Input: part model. Units: mm. Frame: model coordinates. A direction names the side the tool comes from. Give positions to 0.01 mm unless a question says otherwise; leave off trailing zeros. Loops run counter-clockwise (first coordinate to the right, second up) from the corner with the lowest first, then second, coordinate; pieces in that order, holes last. Notation, with made-up numbers: M 0,7.25 L 33,7.25 A14 ccw 33,32.25 Z; hole C 22.25,-8.5 d5. An arc over 180 degrees is marked long. Use CSV: the item, a comma, the result in double quotes. Start each with the question number.
Q1. Reachability of faces 4 (the flat face through (1, 12.573, 6)), 5 (the flat face through (1, 2.286, -1)), 6 (the cylindrical face through (4.34, 46.73, 6.39)) from +Z, -Z, +X, -X, +Y, -Y: full face, straight path, thin tool, end or side. Return the list, or none.
Q2. Section C-C, the plane x = 2. Output: boundary loops of the cut face in (y, z) (3 decimals).
Q3. Pull-direction query (Y, two-part tool) for faces 1 (the cylindrical face through (1.428, 11.809, 9.385)), 2 (the flat face through (18.128, 46, 6)), 3 (the cylindrical face through (1.528, 51.891, 6.386)); classes: released by +Y, released by -Y, zero draft, split by the parting line, or undercut.
Q4. Pin query (flat end, axial travel): pin 1 (0.9 mm diameter, centred on x = 2, z = 7.5, fed in from +Y); pin 2 (8 mm diameter, centred on x = 8.5, y = 11, fed in from -Z); pin 3 (1 mm diameter, centred on x = 1.5, y = 9.5, fed in from -Z); pin 4 (2 mm diameter, centred on x = 9, z = 4, fed in from -Y). Return the tip coordinate at first contact, or that it passes through.
Q5. Section D-D, the plane y = 28. Output: boundary loops of the cut face in (x, z), plus the area to 3 significant figures.
Q6. Section A-A, the plane y = 45.5. Output: boundary loops of the cut face in (x, z), plus the area to 3 significant figures.
Q7. Material intervals for line 1 along Y through (x, z) = (1.5, 5.5) (3 decimals); line 2 along X through (y, z) = (38, 2.5); line 3 along Y through (x, z) = (1, 5.25) (3 decimals), sorted ascending.
Q8. Section B-B, the plane z = 9.25. Output: boundary loops of the cut face in (x, y), plus the area to 3 significant figures.
from build123d import *

# Parameters (mm, degrees)
F1_DEPTH = 12.954
F2_W     = 5.715
F2_H     = 7.2644
F3_DEPTH = 18.129257
F5_DEPTH = 2.8956


with BuildPart() as f1:
    # F0 (on Top) → F1 (new body)
    with BuildSketch(Plane.XY):
        with BuildLine():
            Line((0, 48.26), (0, 0))
            Line((0, 0), (2.8956, 0))
            Line((2.8956, 0), (2.8956, 43.18))
            ThreePointArc((2.8956, 43.18), (4.383498, 46.772102), (7.9756, 48.26))
            Line((7.9756, 48.26), (10.538739, 48.26))
            ThreePointArc((10.538739, 48.26), (13.963674, 46.931829), (15.597704, 43.641818))
            ThreePointArc((15.597704, 43.641818), (15.761106, 43.312817), (16.1036, 43.18))
            Line((16.1036, 43.18), (17.620257, 43.18))
            ThreePointArc((17.620257, 43.18), (17.979467, 43.32879), (18.128257, 43.688))
            Line((18.128257, 43.688), (18.128257, 48.26))
            ThreePointArc((18.128257, 48.26), (16.64036, 51.852102), (13.048257, 53.34))
            Line((13.048257, 53.34), (5.08, 53.34))
            ThreePointArc((5.08, 53.34), (1.487898, 51.852102), (0, 48.26))
        make_face()
    extrude(amount=F1_DEPTH)

    # F2 (on face) → F3 (cut, through all)
    with BuildSketch(Plane(origin=(0, 0, 0), x_dir=(0, -1, 0), z_dir=(-1, 0, 0))):
        with BuildLine():
            ThreePointArc((-15.875, 3.3528), (-15.72621, 2.99359), (-15.367, 2.8448))
            Line((-15.367, 2.8448), (-8.001, 2.8448))
            Line((-8.001, 2.8448), (-8.001, 10.1092))
            Line((-8.001, 10.1092), (-10.033, 10.1092))
            ThreePointArc((-10.033, 10.1092), (-11.829051, 9.365251), (-12.573, 7.5692))
            Line((-12.573, 7.5692), (-12.573, 4.445))
            ThreePointArc((-12.573, 4.445), (-12.72179, 4.08579), (-13.081, 3.937))
            Line((-13.081, 3.937), (-14.351, 3.937))
            ThreePointArc((-14.351, 3.937), (-14.71021, 4.08579), (-14.859, 4.445))
            Line((-14.859, 4.445), (-14.859, 5.842))
            Line((-14.859, 5.842), (-13.97, 5.842))
            Line((-13.97, 5.842), (-13.97, 6.604))
            ThreePointArc((-13.97, 6.604), (-14.11879, 6.96321), (-14.478, 7.112))
            Line((-14.478, 7.112), (-15.367, 7.112))
            ThreePointArc((-15.367, 7.112), (-15.72621, 6.96321), (-15.875, 6.604))
            Line((-15.875, 6.604), (-15.875, 3.3528))
        make_face()
        with Locations((-3.8735, 6.477)):
            Rectangle(F2_W, F2_H)
    extrude(amount=-F3_DEPTH, mode=Mode.SUBTRACT)

    # F4 (on Right) → F5 (join, through all)
    with BuildSketch(Plane.YZ):
        with BuildLine():
            Line((2.286, 0), (0, 0))
            Line((0, 0), (0, -1.524))
            ThreePointArc((0, -1.524), (0.371974, -2.422026), (1.27, -2.794))
            Line((1.27, -2.794), (2.286, -2.794))
            Line((2.286, -2.794), (2.286, 0))
        make_face()
    extrude(amount=F5_DEPTH)


solid = f1.part
A:
1,face 4,"+X, -X"
1,face 5,"-Z, +X, -X, +Y"
1,face 6,"+Z, -Z, -Y"
2,outline,"M 0,-1.524 A1.27 ccw 1.27,-2.794 L 2.286,-2.794 L 2.286,0 L 52.3,0 L 52.3,12.954 L 0,12.954 Z; hole M 1.016,2.845 L 6.731,2.845 L 6.731,10.109 L 1.016,10.109 Z; hole M 8.001,2.845 L 15.367,2.845 A0.508 ccw 15.875,3.353 L 15.875,6.604 A0.508 ccw 15.367,7.112 L 14.478,7.112 A0.508 ccw 13.97,6.604 L 13.97,5.842 L 14.859,5.842 L 14.859,4.445 A0.508 cw 14.351,3.937 L 13.081,3.937 A0.508 cw 12.573,4.445 L 12.573,7.569 A2.54 ccw 10.033,10.109 L 8.001,10.109 Z"
3,face 1,"undercut"
3,face 2,"zero draft"
3,face 3,"released by +Y"
4,pin 1,"y = 52.61"
4,pin 2,"through"
4,pin 3,"z = 0"
4,pin 4,"y = 48.26"
5,outline,"M 0,0 L 2.9,0 L 2.9,12.95 L 0,12.95 Z"
5,area,"37.5 mm^2"
6,outline,"M 0,0 L 3.46,0 L 3.46,12.95 L 0,12.95 Z; M 15.06,0 L 18.13,0 L 18.13,12.95 L 15.06,12.95 Z"
6,area,"84.5 mm^2"
7,line 1,"0 to 1.016, 6.731 to 8.001, 12.573 to 14.859, 15.875 to 51.864"
7,line 2,"0 to 2.9"
7,line 3,"0 to 1.016, 6.731 to 8.001, 12.573 to 14.859, 15.875 to 51.287"
8,outline,"M 0,0 L 2.9,0 L 2.9,1.02 L 0,1.02 Z; M 0,6.73 L 2.9,6.73 L 2.9,8 L 0,8 Z; M 0,11.94 L 2.9,11.94 L 2.9,43.18 A5.08 cw 7.98,48.26 L 10.54,48.26 A5.08 cw 15.6,43.64 A0.51 ccw 16.1,43.18 L 17.62,43.18 A0.51 ccw 18.13,43.69 L 18.13,48.26 A5.08 ccw 13.05,53.34 L 5.08,53.34 A5.08 ccw 0,48.26 Z"
8,area,"217 mm^2"
